Check sheet for the modelled part. Datum: model origin and axes. Units: mm. Face numbers are marked on the shaded views. A direction names the side the tool comes from. Give positions to 0.01 mm unless a question says otherwise; leave off trailing zeros. Order: outer loops, then holes, each group sorted by start corner. A loop starts at its lowest first (then second) coordinate and runs counter-clockwise, first axis right, second up.
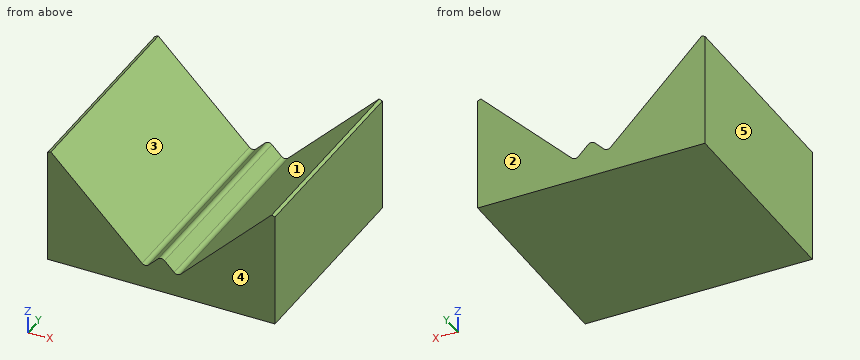
```python
from build123d import *

# Parameters (mm, degrees)
F1_DEPTH = 4.6
F2_SIZE  = 0.2
F3_SIZE  = 0.2
F4_R     = 0.2


with BuildPart() as f1:
    # F0 (on Front) → F1 (new body, symmetric)
    with BuildSketch(Plane.XZ):
        Polygon((0, 5.228932), (0, 0), (10, 0), (10, 5.228932), (9.313961, 4.542893), (5.707107, 0.936039), (5, 1.643146), (4.292893, 0.936039), (0.686039, 4.542893), align=None)
    extrude(amount=F1_DEPTH, both=True)

    # F2
    f2_edges = [f1.edges().sort_by_distance(p)[0] for p in [
        (0, 0, 5.228932),
    ]]
    chamfer(f2_edges, length=F2_SIZE)

    # F3
    f3_edges = [f1.edges().sort_by_distance(p)[0] for p in [
        (10, 0, 5.228932),
    ]]
    chamfer(f3_edges, length=F3_SIZE)

    # F4
    f4_edges = [f1.edges().sort_by_distance(p)[0] for p in [
        (4.292893, 0, 0.936039),
        (5, 0, 1.643146),
        (5.707107, 0, 0.936039),
    ]]
    fillet(f4_edges, radius=F4_R)


solid = f1.part
```
Q1. Tool access check on the marked faces 1 and 2. Record the directions out of +Z, -Z, +X, -X, +Y, -Y that give a thin tool (end or side, any length) a straight path to the whole face; none if there is none.
Q2. Sectioned sample at C-C, the plane x = 5. Record the cut outline in (y, z).
Q3. Sectioned sample at A-A, the plane y = 0. Record the cut outline in (x, z), plus the area to 3 significant figures.
Q4. Sectioned sample at B-B, the plane z = 3.6. Record the cut outline in (x, y), plus the area to 3 significant figures.
Q5. Material ranges on line 1 (X direction, y = 1.75, z = 2.9); line 2 (X direction, y = 4, z = 1.3); line 3 (X direction, y = -2.25, z = 2.55), recorded low to high.
Q6. Draft check along X on the marked faces 3, 4 and 5. Enter one of: pulls with the +X half, pulls with the -X half, needs draft (parallel to the pull), parting line crosses it, or undercut.
Q7. Sectioned sample at D-D, the plane z = 4.35. Record the cut outline in (x, y), plus the area to 3 significant figures.
Q8. Go/stop test with flat-tipped pins: P1, Ø1, axis at x = 5, y = 0, coming from the +Z side; P2, Ø5, axis at x = 4.5, y = 0, coming from the +Z side. Record where each tip stops, or that it passes through.
Filled in:
1. face 1: +Z, +Y, -Y
1. face 2: +Z, -Z, +X, -X, +Y
2. outline: (-4.6, 0) - (4.6, 0) - (4.6, 1.56) - (-4.6, 1.56) - close
3. outline: (0, 0) - (10, 0) - (10, 5.03) - (9.86, 5.09) - (5.85, 1.08) arc R0.2 cw to (5.57, 1.08) - (5.14, 1.5) arc R0.2 ccw to (4.86, 1.5) - (4.43, 1.08) arc R0.2 cw to (4.15, 1.08) - (0.14, 5.09) - (0, 5.03) - close
3. area: 28.3 mm2
4. outline: (0, -4.6) - (1.63, -4.6) - (1.63, 4.6) - (0, 4.6) - close; (8.37, -4.6) - (10, -4.6) - (10, 4.6) - (8.37, 4.6) - close
4. area: 30.0 mm2
5. line 1: x = 0 to 2.33, 7.67 to 10
5. line 2: x = 0 to 3.93, 4.66 to 5.34, 6.07 to 10
5. line 3: x = 0 to 2.68, 7.32 to 10
6. face 3: undercut
6. face 4: needs draft
6. face 5: pulls with the -X half
7. outline: (0, -4.6) - (0.88, -4.6) - (0.88, 4.6) - (0, 4.6) - close; (9.12, -4.6) - (10, -4.6) - (10, 4.6) - (9.12, 4.6) - close
7. area: 16.2 mm2
8. P1: stops at z = 1.56
8. P2: stops at z = 3.23
